Build history of the part. All positions in model axes, mm. A direction names the side the tool comes from. Coordinates: 2 decimals unless noted, no trailing zeros. Loops run counter-clockwise (first coordinate to the right, second up) from the corner with the lowest first, then second, coordinate; pieces in that order, holes last. Notation, with made-up numbers: (79, -35) - (119, -35) arc R20 ccw to (119, -3) - close; hole circle Ø1 at (-40, 66). An arc over 180 degrees is marked (long way). One line per item, written item: value.
```python
from build123d import *

# Parameters (mm, degrees)
SKETCH1_W           = 89.2
SKETCH1_H           = 28
BOSS_EXTRUDE1_DEPTH = 2
SKETCH3_W           = 89.2
SKETCH3_H           = 28
SKETCH3_W_2         = 85.2
SKETCH3_H_2         = 24
BOSS_EXTRUDE2_DEPTH = 1.5
CUT_EXTRUDE1_REACH  = 48.788
SKETCH5_W           = 7
SKETCH5_H           = 4.35
BOSS_EXTRUDE3_DEPTH = 5
SKETCH6_R           = 1
CUT_EXTRUDE2_DEPTH  = 54.124005873
BOSS_EXTRUDE4_DEPTH = 4.35
BOSS_EXTRUDE5_DEPTH = 4.35
CHAMFER1_SIZE       = 1.2
CHAMFER2_SIZE       = 1.2
SKETCH9_W           = 6.7
SKETCH9_H           = 6.85
BOSS_EXTRUDE6_DEPTH = 1.5
SKETCH15_W          = 6.7
SKETCH15_H          = 1.6
BOSS_EXTRUDE7_DEPTH = 8.3
CUT_EXTRUDE9_REACH  = 55.565
SKETCH16_R          = 0.925
CUT_EXTRUDE11_REACH = 55.565
SKETCH17_R          = 0.9
CHAMFER3_SIZE       = 1.2
CHAMFER4_SIZE       = 1.2
CUT_EXTRUDE12_DEPTH = 48.76190951
CHAMFER5_SIZE       = 0.5
CHAMFER6_SIZE       = 0.5


with BuildPart() as part:
    # Sketch1 → Boss-Extrude1 (new body)
    with BuildSketch(Plane(origin=(0, 0, 0), x_dir=(1, 0, 0), z_dir=(0, 1, 0))):
        Rectangle(SKETCH1_W, SKETCH1_H)
    extrude(amount=BOSS_EXTRUDE1_DEPTH)

    # Sketch3 → Boss-Extrude2 (add)
    with BuildSketch(Plane.XZ):
        Rectangle(SKETCH3_W, SKETCH3_H)
        Rectangle(SKETCH3_W_2, SKETCH3_H_2, mode=Mode.SUBTRACT)
    extrude(amount=BOSS_EXTRUDE2_DEPTH)

    # Sketch4 → Cut-Extrude1 (cut, up to next)
    with BuildSketch(Plane.XZ, mode=Mode.PRIVATE) as cut_extrude1_sk1:
        Polygon((38.6, -8), (38.6, 8), (29.362395693, -8), align=None)
    cut_extrude1_tool1 = extrude(cut_extrude1_sk1.sketch, amount=-CUT_EXTRUDE1_REACH, mode=Mode.PRIVATE) & part.part
    # Sketch4 → Cut-Extrude1 (cut, up to next)
    with BuildSketch(Plane.XZ, mode=Mode.PRIVATE) as cut_extrude1_sk2:
        Polygon((35.135898385, 8), (3.464101615, 8), (12.701705922, -8), (25.898294078, -8), align=None)
    cut_extrude1_tool2 = extrude(cut_extrude1_sk2.sketch, amount=-CUT_EXTRUDE1_REACH, mode=Mode.PRIVATE) & part.part
    # Sketch4 → Cut-Extrude1 (cut, up to next)
    with BuildSketch(Plane.XZ, mode=Mode.PRIVATE) as cut_extrude1_sk3:
        Polygon((-38.6, 8), (-38.6, -8), (-29.362395693, -8), align=None)
    cut_extrude1_tool3 = extrude(cut_extrude1_sk3.sketch, amount=-CUT_EXTRUDE1_REACH, mode=Mode.PRIVATE) & part.part
    # Sketch4 → Cut-Extrude1 (cut, up to next)
    with BuildSketch(Plane.XZ, mode=Mode.PRIVATE) as cut_extrude1_sk4:
        Polygon((0, 8), (-9.237604307, -8), (9.237604307, -8), align=None)
    cut_extrude1_tool4 = extrude(cut_extrude1_sk4.sketch, amount=-CUT_EXTRUDE1_REACH, mode=Mode.PRIVATE) & part.part
    # Sketch4 → Cut-Extrude1 (cut, up to next)
    with BuildSketch(Plane.XZ, mode=Mode.PRIVATE) as cut_extrude1_sk5:
        Polygon((-3.464101615, 8), (-12.701705922, -8), (-25.898294078, -8), (-35.135898385, 8), align=None)
    cut_extrude1_tool5 = extrude(cut_extrude1_sk5.sketch, amount=-CUT_EXTRUDE1_REACH, mode=Mode.PRIVATE) & part.part
    add(cut_extrude1_tool1.solids().sort_by_distance((35.520799, 0, -2.666667))[0], mode=Mode.SUBTRACT)
    add(cut_extrude1_tool2.solids().sort_by_distance((19.3, 0, 1.098039))[0], mode=Mode.SUBTRACT)
    add(cut_extrude1_tool3.solids().sort_by_distance((-35.520799, 0, -2.666667))[0], mode=Mode.SUBTRACT)
    add(cut_extrude1_tool4.solids().sort_by_distance((0, 0, -2.666667))[0], mode=Mode.SUBTRACT)
    add(cut_extrude1_tool5.solids().sort_by_distance((-19.3, 0, 1.098039))[0], mode=Mode.SUBTRACT)

    # Sketch5 → Boss-Extrude3 (add)
    with BuildSketch(Plane(origin=(0, 2, 0), x_dir=(1, 0, 0), z_dir=(0, 1, 0))):
        with Locations((0, 11.825)):
            Rectangle(SKETCH5_W, SKETCH5_H)
        with Locations((0, -11.825)):
            Rectangle(SKETCH5_W, SKETCH5_H)
    extrude(amount=BOSS_EXTRUDE3_DEPTH)

    # Sketch6 → Cut-Extrude2 (cut, through all)
    with BuildSketch(Plane.XY.offset(14)):
        with Locations((0, 4)):
            Circle(SKETCH6_R)
    extrude(amount=-CUT_EXTRUDE2_DEPTH, mode=Mode.SUBTRACT)

    # Sketch7 → Boss-Extrude4 (add)
    with BuildSketch(Plane.XY.offset(14)):
        Polygon((3.5, 7), (3.5, 2), (15.5, 2), align=None)
        Polygon((-3.5, 7), (-3.5, 2), (-15.5, 2), align=None)
    extrude(amount=-BOSS_EXTRUDE4_DEPTH)

    # Sketch8 → Boss-Extrude5 (add)
    with BuildSketch(Plane(origin=(0, 0, -14), x_dir=(-1, 0, 0), z_dir=(0, 0, -1))):
        Polygon((3.5, 7), (3.5, 2), (15.5, 2), align=None)
        Polygon((-3.5, 7), (-3.5, 2), (-15.5, 2), align=None)
    extrude(amount=-BOSS_EXTRUDE5_DEPTH)

    # Chamfer1
    chamfer1_edges = [part.edges().sort_by_distance(p)[0] for p in [
        (-1, 4, -14),
    ]]
    chamfer(chamfer1_edges, length=CHAMFER1_SIZE)

    # Chamfer2
    chamfer2_edges = [part.edges().sort_by_distance(p)[0] for p in [
        (-1, 4, 14),
    ]]
    chamfer(chamfer2_edges, length=CHAMFER2_SIZE)

    # Sketch9 → Boss-Extrude6 (add)
    with BuildSketch(Plane.XY.offset(14)):
        with Locations((0, -4.925)):
            Rectangle(SKETCH9_W, SKETCH9_H)
    extrude(amount=-BOSS_EXTRUDE6_DEPTH)

    # Sketch15 → Boss-Extrude7 (add)
    with BuildSketch(Plane.XZ.offset(1.5)):
        with Locations((14.5, -13.2)):
            Rectangle(SKETCH15_W, SKETCH15_H)
        with Locations((-14.5, -13.2)):
            Rectangle(SKETCH15_W, SKETCH15_H)
    extrude(amount=BOSS_EXTRUDE7_DEPTH)

    # Sketch16 → Cut-Extrude9 (cut, up to next)
    with BuildSketch(Plane(origin=(0, 0, -14), x_dir=(-1, 0, 0), z_dir=(0, 0, -1)), mode=Mode.PRIVATE) as cut_extrude9_sk1:
        with Locations((14.5, -7.35)):
            Circle(SKETCH16_R)
    cut_extrude9_tool1 = extrude(cut_extrude9_sk1.sketch, amount=-CUT_EXTRUDE9_REACH, mode=Mode.PRIVATE) & part.part
    # Sketch16 → Cut-Extrude9 (cut, up to next)
    with BuildSketch(Plane(origin=(0, 0, -14), x_dir=(-1, 0, 0), z_dir=(0, 0, -1)), mode=Mode.PRIVATE) as cut_extrude9_sk2:
        with Locations((-14.5, -7.35)):
            Circle(SKETCH16_R)
    cut_extrude9_tool2 = extrude(cut_extrude9_sk2.sketch, amount=-CUT_EXTRUDE9_REACH, mode=Mode.PRIVATE) & part.part
    add(cut_extrude9_tool1.solids().sort_by_distance((-14.5, -7.35, -14))[0], mode=Mode.SUBTRACT)
    add(cut_extrude9_tool2.solids().sort_by_distance((14.5, -7.35, -14))[0], mode=Mode.SUBTRACT)

    # Sketch17 → Cut-Extrude11 (cut, up to next)
    with BuildSketch(Plane.XY.offset(14), mode=Mode.PRIVATE) as cut_extrude11_sk1:
        with Locations((0.155335946, -6.45)):
            Circle(SKETCH17_R)
    cut_extrude11_tool1 = extrude(cut_extrude11_sk1.sketch, amount=-CUT_EXTRUDE11_REACH, mode=Mode.PRIVATE) & part.part
    add(cut_extrude11_tool1.solids().sort_by_distance((0.155336, -6.45, 14))[0], mode=Mode.SUBTRACT)

    # Chamfer3
    # the kernel refuses this chamfer: 1.2 mm, written as the material it takes off along each edge
    with BuildSketch(Plane(origin=(0.155335946, -6.45, 14), x_dir=(1, 0, 0), z_dir=(0, -1, 0))) as chamfer3_piece_1:
        Polygon((0.9 + CHAMFER3_SIZE, 0), (0.9, -CHAMFER3_SIZE), (0.9, 0), align=None)
    revolve(axis=Axis((0.155335946, -6.45, 14), (0, 0, 1)), mode=Mode.SUBTRACT)

    # Chamfer4
    chamfer4_edges = [part.edges().sort_by_distance(p)[0] for p in [
        (-13.575, -7.35, -14),
        (15.425, -7.35, -14),
    ]]
    chamfer(chamfer4_edges, length=CHAMFER4_SIZE)

    # Sketch18 → Cut-Extrude12 (cut, through all)
    with BuildSketch(Plane.XZ):
        with BuildLine():
            Line((38.6, 3.26), (38.6, 8))
            ThreePointArc((38.6, 8), (40.97, 5.63), (38.6, 3.26))
        make_face()
        with BuildLine():
            Line((-38.6, 8), (-38.6, 3.257907009))
            ThreePointArc((-38.6, 3.257907009), (-40.971046495, 5.628953505), (-38.6, 8))
        make_face()
    extrude(amount=-CUT_EXTRUDE12_DEPTH, mode=Mode.SUBTRACT)

    # Chamfer5
    chamfer5_edges = [part.edges().sort_by_distance(p)[0] for p in [
        (0, 7, -9.65),
        (-9.5, 4.5, -9.65),
        (9.5, 4.5, -9.65),
    ]]
    chamfer(chamfer5_edges, length=CHAMFER5_SIZE)

    # Chamfer6
    chamfer6_edges = [part.edges().sort_by_distance(p)[0] for p in [
        (0, 7, 9.65),
        (9.5, 4.5, 9.65),
        (-9.5, 4.5, 9.65),
    ]]
    chamfer(chamfer6_edges, length=CHAMFER6_SIZE)


solid = part.part
```
Item 1: Cut at B-B, the plane z = -4. Write the cut outline in (x, y).
Check result:
outline: (-44.6, -1.5) - (-42.6, -1.5) - (-42.6, 0) - (-38.6, 0) - (-38.6, 2) - (-44.6, 2) - close; (-31.67, 0) - (-28.21, 0) - (-28.21, 2) - (-31.67, 2) - close; (-10.39, 0) - (-6.93, 0) - (-6.93, 2) - (-10.39, 2) - close; (6.93, 0) - (10.39, 0) - (10.39, 2) - (6.93, 2) - close; (28.21, 0) - (31.67, 0) - (31.67, 2) - (28.21, 2) - close; (38.6, 0) - (42.6, 0) - (42.6, -1.5) - (44.6, -1.5) - (44.6, 2) - (38.6, 2) - close
Item 2: Cut at D-D, the plane z = 7. Write the cut outline in (x, y).
Check result:
outline: (-44.6, -1.5) - (-42.6, -1.5) - (-42.6, 0) - (-40.53, 0) - (-40.53, 2) - (-44.6, 2) - close; (-38.02, 0) - (-34.56, 0) - (-34.56, 2) - (-38.02, 2) - close; (-4.04, 0) - (-0.58, 0) - (-0.58, 2) - (-4.04, 2) - close; (0.58, 0) - (4.04, 0) - (4.04, 2) - (0.58, 2) - close; (34.56, 0) - (38.02, 0) - (38.02, 2) - (34.56, 2) - close; (40.53, 0) - (42.6, 0) - (42.6, -1.5) - (44.6, -1.5) - (44.6, 2) - (40.53, 2) - close
Item 3: Tool access for faces 4 (the face through (-19, 1, -8)), 5 (the face through (-9.487, 4.231, -9.896)), 6 (the face through (0.2, 2.8, -9.65)), 7 (the face through (-0.6, 2, -9.5)), 8 (the face through (-42.6, -1, 0)): list every direction of +Z, -Z, +X, -X, +Y, -Y with a clear straight run to the whole face (end or side of a thin tool).
Check result:
face 4: +Y, -Y
face 5: -X, +Y
face 6: +X, -X, +Y
face 7: +Y
face 8: -Y
Item 4: Probe probe 1 along Z at (x, y) = (-34, 1); probe 2 along X at (y, z) = (1.25, -0.75); probe 3 along Z at (x, y) = (17.5, -8). List the from-to ranges inside material, lowest first. Write a range as from..to.
Check result:
probe 1: z = -14..-8, 0.03..6.03, 8..14
probe 2: x = -44.6..-38.6, -33.55..-30.08, -8.52..-5.05, 5.05..8.52, 30.08..33.55, 38.6..44.6
probe 3: z = -14..-12.4
Item 5: Drop flat-ended pins along their axis: P1, Ø12, axis at x = 35, z = 10.5, coming from the +Y side; P2, Ø0.8, axis at x = -1.5, z = 13, coming from the -Y side; P3, Ø2.5, axis at x = 14.5, y = -7.35, coming from the -Z side (3 decimals). Give the stop position or say it passes through.
Check result:
P1: stops at y = 2
P2: stops at y = -8.35
P3: stops at z = -13.125
Item 6: Cut at A-A, the plane y = 4. Write the cut outline in (x, z), then the cut area to 3 significant figures.
Check result:
outline: (-10.7, -14) - (-2.2, -14) - (-1, -12.8) - (-1, -9.65) - (-9.4, -9.65) - (-10.7, -10.15) - close; (-10.7, 10.15) - (-9.4, 9.65) - (-1, 9.65) - (-1, 12.8) - (-2.2, 14) - (-10.7, 14) - close; (1, -12.8) - (2.2, -14) - (10.7, -14) - (10.7, -10.15) - (9.4, -9.65) - (1, -9.65) - close; (1, 9.65) - (9.4, 9.65) - (10.7, 10.15) - (10.7, 14) - (2.2, 14) - (1, 12.8) - close
area: 165 mm^2
Item 7: Cut at C-C, the plane x = 31.5. Write the cut outline in (y, z).
Check result:
outline: (-1.5, -14) - (2, -14) - (2, -8) - (0, -8) - (0, -12) - (-1.5, -12) - close; (-1.5, 12) - (0, 12) - (0, 8) - (2, 8) - (2, 14) - (-1.5, 14) - close; (0, -4.3) - (2, -4.3) - (2, 1.7) - (0, 1.7) - close
Item 8: Pull direction X, two halves, no side cores. Call faces 1 (the face through (0, 7, -12)), 2 (the face through (8.02, 0.99, 0.11)), 3 (the face through (-17.85, -6, -13)): released by +X, released by -X, zero draft, split by the parting line, or undercut.
Check result:
face 1: zero draft
face 2: undercut
face 3: released by -X
